Could you check a few things on this model? Use its own coordinates, in mm. Round coordinates to 2 decimals unless told otherwise and drop trailing zeros. Write each loop counter-clockwise with the first axis right and the second up, starting at its lowest first coordinate (ties: lowest second). Pieces come first, ordered by that corner, then holes. Notation, with made-up numbers: (86.25, 89) -> (104.25, 89) arc R21 ccw to (104.25, 94) -> close; hole circle Ø8 at (-24.75, 8). An arc over 180 degrees is marked (long way). Answer in a Markdown table with one row per item. Add a question column.
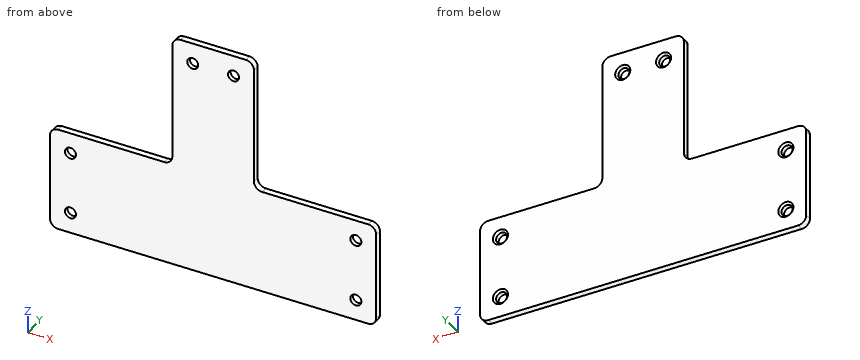
```python
from build123d import *

# Parameters (mm, degrees)
SKETCH1_W           = 80
SKETCH1_H           = 25
BOSS_EXTRUDE1_DEPTH = 1.6
SKETCH2_W           = 20
SKETCH2_H           = 32
BOSS_EXTRUDE2_DEPTH = 1.6
SKETCH3_R           = 1.35
CUT_EXTRUDE1_DEPTH  = 1.6
SKETCH4_R           = 1.35
CUT_EXTRUDE2_DEPTH  = 1.6
SKETCH5_R           = 1.35
CUT_EXTRUDE3_DEPTH  = 1.6
SKETCH6_R           = 1.35
CUT_EXTRUDE4_DEPTH  = 1.6
SKETCH7_R           = 1.35
CUT_EXTRUDE5_DEPTH  = 1.6
SKETCH8_R           = 1.35
CUT_EXTRUDE6_DEPTH  = 1.6
CHAMFER1_SIZE       = 0.5
FILLET1_R           = 2


with BuildPart() as part:
    # Sketch1 → Boss-Extrude1 (new body)
    with BuildSketch(Plane(origin=(0, 0, 0), x_dir=(1, 0, 0), z_dir=(0, 1, 0))):
        Rectangle(SKETCH1_W, SKETCH1_H)
    extrude(amount=BOSS_EXTRUDE1_DEPTH)

    # Sketch2 → Boss-Extrude2 (add)
    with BuildSketch(Plane(origin=(0, 1.6, 0), x_dir=(1, 0, 0), z_dir=(0, 1, 0))):
        with Locations((0, -28.5)):
            Rectangle(SKETCH2_W, SKETCH2_H)
    extrude(amount=-BOSS_EXTRUDE2_DEPTH)

    # Sketch3 → Cut-Extrude1 (cut)
    with BuildSketch(Plane(origin=(0, 1.6, 0), x_dir=(1, 0, 0), z_dir=(0, 1, 0))):
        with Locations(Location((-35, 7.5, 0), (0, 0, 270))):
            Circle(SKETCH3_R)
    extrude(amount=-CUT_EXTRUDE1_DEPTH, mode=Mode.SUBTRACT)

    # Sketch4 → Cut-Extrude2 (cut)
    with BuildSketch(Plane(origin=(0, 1.6, 0), x_dir=(1, 0, 0), z_dir=(0, 1, 0))):
        with Locations(Location((35, 7.5, 0), (0, 0, 270))):
            Circle(SKETCH4_R)
    extrude(amount=-CUT_EXTRUDE2_DEPTH, mode=Mode.SUBTRACT)

    # Sketch5 → Cut-Extrude3 (cut)
    with BuildSketch(Plane(origin=(0, 1.6, 0), x_dir=(1, 0, 0), z_dir=(0, 1, 0))):
        with Locations(Location((-35, -7.5, 0), (0, 0, 270))):
            Circle(SKETCH5_R)
    extrude(amount=-CUT_EXTRUDE3_DEPTH, mode=Mode.SUBTRACT)

    # Sketch6 → Cut-Extrude4 (cut)
    with BuildSketch(Plane(origin=(0, 1.6, 0), x_dir=(1, 0, 0), z_dir=(0, 1, 0))):
        with Locations(Location((35, -7.5, 0), (0, 0, 270))):
            Circle(SKETCH6_R)
    extrude(amount=-CUT_EXTRUDE4_DEPTH, mode=Mode.SUBTRACT)

    # Sketch7 → Cut-Extrude5 (cut)
    with BuildSketch(Plane(origin=(0, 1.6, 0), x_dir=(1, 0, 0), z_dir=(0, 1, 0))):
        with Locations(Location((-5, -39.5, 0), (0, 0, 270))):
            Circle(SKETCH7_R)
    extrude(amount=-CUT_EXTRUDE5_DEPTH, mode=Mode.SUBTRACT)

    # Sketch8 → Cut-Extrude6 (cut)
    with BuildSketch(Plane(origin=(0, 1.6, 0), x_dir=(1, 0, 0), z_dir=(0, 1, 0))):
        with Locations(Location((5, -39.5, 0), (0, 0, 270))):
            Circle(SKETCH8_R)
    extrude(amount=-CUT_EXTRUDE6_DEPTH, mode=Mode.SUBTRACT)

    # Chamfer1
    chamfer1_edges = [part.edges().sort_by_distance(p)[0] for p in [
        (-35, 1.6, -8.85),
        (35, 1.6, -8.85),
        (-35, 1.6, 6.15),
        (35, 1.6, 6.15),
        (-5, 1.6, 38.15),
        (5, 1.6, 38.15),
    ]]
    chamfer(chamfer1_edges, length=CHAMFER1_SIZE)

    # Fillet1
    fillet1_edges = [part.edges().sort_by_distance(p)[0] for p in [
        (-40, 0.8, -12.5),
        (40, 0.8, -12.5),
        (40, 0.8, 12.5),
        (10, 0.8, 12.5),
        (10, 0.8, 44.5),
        (-10, 0.8, 44.5),
        (-10, 0.8, 12.5),
        (-40, 0.8, 12.5),
    ]]
    fillet(fillet1_edges, radius=FILLET1_R)


solid = part.part
```
(1) I need wall thicknesses on L1, parallel to X at y = 0.8, z = 39.5; L2, parallel to X at y = 0.7, z = 7.5; L3, parallel to X at y = 0.5, z = 32. Which ranges of each line are inside material? Lowest first, please.
(2) Suppose I cut it at D-D, the plane y = 0.65. Please give me the cut outline in (x, z).
(3) Suppose I cut it at B-B, the plane z = -7.5. Please give me the cut outline in (x, y), then the cut area to 3 significant figures.
(4) Suppose I cut it at C-C, the plane x = -5. Please give me the cut outline in (y, z).
(5) For P1, Ø0.8, axis at y = 0.5, z = 30.5, coming from the -X side; P2, Ø0.8, axis at x = -28.5, y = 1, coming from the +Z side; P3, Ø3, axis at x = -35, z = 7.5, coming from the +Y side, each with a flat end and sliding along its axis, tell me the tip position at first contact or that it passes through.
(6) Suppose I cut it at A-A, the plane x = -35. Please give me the cut outline in (y, z).
Response:
| question | item | result |
|---|---|---|
| 1 | L1 | -10 to -6.35, -3.65 to 3.65, 6.35 to 10 |
| 1 | L2 | -40 to -36.35, -33.65 to 33.65, 36.35 to 40 |
| 1 | L3 | -10 to 10 |
| 2 | outline | (-40, -10.5) arc R2 ccw to (-38, -12.5) -> (38, -12.5) arc R2 ccw to (40, -10.5) -> (40, 10.5) arc R2 ccw to (38, 12.5) -> (12, 12.5) arc R2 cw to (10, 14.5) -> (10, 42.5) arc R2 ccw to (8, 44.5) -> (-8, 44.5) arc R2 ccw to (-10, 42.5) -> (-10, 14.5) arc R2 cw to (-12, 12.5) -> (-38, 12.5) arc R2 ccw to (-40, 10.5) -> close; hole circle Ø2.7 at (-35, -7.5); hole circle Ø2.7 at (-35, 7.5); hole circle Ø2.7 at (-5, 39.5); hole circle Ø2.7 at (5, 39.5); hole circle Ø2.7 at (35, -7.5); hole circle Ø2.7 at (35, 7.5) |
| 3 | outline | (-40, 0) -> (-36.35, 0) -> (-36.35, 1.1) -> (-36.85, 1.6) -> (-40, 1.6) -> close; (-33.65, 0) -> (33.65, 0) -> (33.65, 1.1) -> (33.15, 1.6) -> (-33.15, 1.6) -> (-33.65, 1.1) -> close; (36.35, 0) -> (40, 0) -> (40, 1.6) -> (36.85, 1.6) -> (36.35, 1.1) -> close |
| 3 | area | 119 mm² |
| 4 | outline | (0, -12.5) -> (1.6, -12.5) -> (1.6, 37.65) -> (1.1, 38.15) -> (0, 38.15) -> close; (0, 40.85) -> (1.1, 40.85) -> (1.6, 41.35) -> (1.6, 44.5) -> (0, 44.5) -> close |
| 5 | P1 | x = -10 |
| 5 | P2 | z = 12.5 |
| 5 | P3 | y = 1.25 |
| 6 | outline | (0, -12.5) -> (1.6, -12.5) -> (1.6, -9.35) -> (1.1, -8.85) -> (0, -8.85) -> close; (0, -6.15) -> (1.1, -6.15) -> (1.6, -5.65) -> (1.6, 5.65) -> (1.1, 6.15) -> (0, 6.15) -> close; (0, 8.85) -> (1.1, 8.85) -> (1.6, 9.35) -> (1.6, 12.5) -> (0, 12.5) -> close |
